```python
from build123d import *

# Parameters (mm, degrees)
SKETCH1_W           = 5
SKETCH1_H           = 5
BOSS_EXTRUDE1_DEPTH = 110
SKETCH2_W           = 3
SKETCH2_H           = 3
CUT_EXTRUDE1_DEPTH  = 9
SKETCH3_W           = 3
SKETCH3_H           = 3
CUT_EXTRUDE2_DEPTH  = 9


with BuildPart() as part:
    # Sketch1 → Boss-Extrude1 (new body)
    with BuildSketch(Plane.XY):
        with Locations((2.5, 2.5)):
            Rectangle(SKETCH1_W, SKETCH1_H)
    extrude(amount=BOSS_EXTRUDE1_DEPTH)

    # Sketch2 → Cut-Extrude1 (cut)
    with BuildSketch(Plane.ZY):
        with Locations((2.5, 2.5)):
            Rectangle(SKETCH2_W, SKETCH2_H)
        with Locations((107.5, 2.5)):
            Rectangle(SKETCH2_W, SKETCH2_H)
    extrude(amount=-CUT_EXTRUDE1_DEPTH, mode=Mode.SUBTRACT)

    # Sketch3 → Cut-Extrude2 (cut)
    with BuildSketch(Plane(origin=(0, 5, 0), x_dir=(1, 0, 0), z_dir=(0, 1, 0))):
        with Locations((2.5, -25.15)):
            Rectangle(SKETCH3_W, SKETCH3_H)
    extrude(amount=-CUT_EXTRUDE2_DEPTH, mode=Mode.SUBTRACT)


solid = part.part
```
Design review of the part built by this model. Coordinates are the model's own, in mm. A direction names the side the tool comes from. Give positions to 0.01 mm unless a question says otherwise; leave off trailing zeros. Write each loop counter-clockwise with the first axis right and the second up, starting at its lowest first coordinate (ties: lowest second). Pieces come first, ordered by that corner, then holes. Notation, with made-up numbers: (3.5, 78.25) - (15.5, 78.25) arc R11 cw to (15.5, 98.25) - close; hole circle Ø10 at (-16, 35). An arc over 180 degrees is marked (long way). Return JSON: item names as keys, results as strings. Group by question number.
(1) Machinability: for faces 1 (the flat face through (2, 3, 26.65)), 2 (the flat face through (2, 3, 110)), 3 (the flat face through (2, 2, 1)), which of the approach directions +Z, -Z, +X, -X, +Y, -Y give a long, thin tool a straight path to every point of the face, cutting with its end or side? Answer none if there is none.
(2) Insertion check: pin 1 (1.5 mm diameter, centred on y = 2.5, z = 32, fed in from -X). The pin has a flat end and moves straight along its axis. Give the tip position at first contact, or say it passes through.
(3) We need section A-A, the plane x = 2.15. Give the boundary of the cut face in (y, z).
(4) We need section B-B, the plane y = 2. Give the boundary of the cut face in (x, z).
(5) To check wall thickness, follow probe 1 along Z at (x, y) = (0.65, 3.35); probe 2 along Z at (x, y) = (1.2, 3.4); probe 3 along Z at (x, y) = (2.05, 0.4). State the ranges of each line that lie inside material, in increasing order.
(6) Mouldability with a two-part tool opening along X and no side actions: class faces 4 (the flat face through (5, 2, 54)), 5 (the flat face through (1, 3, 25)), 6 (the flat face through (2, 3, 23.65)), 7 (the flat face through (2, 2, 109)) as +X half, -X half, draft (parallel to the pull), parting line (faces both ways), or undercut.
Reported:
{
 "1": {"face 1": "+Y, -Y", "face 2": "+Z, +X, -X, +Y, -Y", "face 3": "+X, -X"},
 "2": {"pin 1": "stops at x = 0"},
 "3": {"outline": "(0, 0) - (5, 0) - (5, 23.65) - (0, 23.65) - close; (0, 26.65) - (5, 26.65) - (5, 110) - (0, 110) - close; hole (1, 1) - (4, 1) - (4, 4) - (1, 4) - close; hole (1, 106) - (4, 106) - (4, 109) - (1, 109) - close"},
 "4": {"outline": "(0, 0) - (5, 0) - (5, 1) - (0, 1) - close; (0, 4) - (5, 4) - (5, 106) - (0, 106) - close; (0, 109) - (5, 109) - (5, 110) - (0, 110) - close; hole (1, 23.65) - (4, 23.65) - (4, 26.65) - (1, 26.65) - close"},
 "5": {"probe 1": "z = 0 to 1, 4 to 106, 109 to 110", "probe 2": "z = 0 to 1, 4 to 23.65, 26.65 to 106, 109 to 110", "probe 3": "z = 0 to 23.65, 26.65 to 110"},
 "6": {"face 4": "+X half", "face 5": "undercut", "face 6": "undercut", "face 7": "draft"}
}
